```python
from build123d import *

# Parameters (mm, degrees)
BOSS_EXTRUDE1_START = -4
BOSS_EXTRUDE1_DEPTH = 8
CUT_EXTRUDE1_START  = -8
CUT_EXTRUDE1_DEPTH  = 6.4
CUT_EXTRUDE2_DEPTH  = 22.959710978
FILLET1_R           = 2.54
SKETCH6_R           = 3.25
CUT_EXTRUDE5_DEPTH  = 6.80625
LPATTERN1_COUNT     = 4
LPATTERN1_PITCH     = 8
SKETCH4_R           = 1.651
CUT_EXTRUDE3_DEPTH  = 36.358576134
SKETCH5_R           = 3.175
CUT_EXTRUDE4_DEPTH  = 2.54


# Read off the part's stored shape, not the designer's step: Boss-Extrude1
with BuildPart() as part:
    # Boss-Extrude1 outline → Boss-Extrude1 (new body)
    with BuildSketch(Plane(origin=(0, 0, 0), x_dir=(1, 0, 0), z_dir=(0, 1, 0)).offset(BOSS_EXTRUDE1_START)):
        Polygon((0, -4.7625), (0, 0), (-7.9375, 0), (-7.9375, 12.7), (-17.4625, 12.7), (-17.4625, -4.7625), align=None)
    extrude(amount=BOSS_EXTRUDE1_DEPTH)

    # Sketch2 → Cut-Extrude1 (cut)
    with BuildSketch(Plane(origin=(0, 0, -12.7), x_dir=(-1, 0, 0), z_dir=(0, 0, -1)).offset(CUT_EXTRUDE1_START)):
        with BuildLine():
            Line((17.4625, -3.1), (12.625, -3.1))
            ThreePointArc((12.625, -3.1), (9.525, 0), (12.625, 3.1))
            Line((12.625, 3.1), (17.4625, 3.1))
            ThreePointArc((17.4625, 3.1), (20.5625, 0), (17.4625, -3.1))
        make_face()
    extrude(amount=-CUT_EXTRUDE1_DEPTH, mode=Mode.SUBTRACT)

    # Sketch3 → Cut-Extrude2 (cut, through all)
    with BuildSketch(Plane.ZY.offset(17.4625)):
        with BuildLine():
            Line((-12.7, 0.79375), (-5.89375, 0.79375))
            ThreePointArc((-5.89375, 0.79375), (-5.1, 0), (-5.89375, -0.79375))
            Line((-5.89375, -0.79375), (-12.7, -0.79375))
            ThreePointArc((-12.7, -0.79375), (-13.49375, 0), (-12.7, 0.79375))
        make_face()
    extrude(amount=-CUT_EXTRUDE2_DEPTH, mode=Mode.SUBTRACT)

    # Fillet1
    fillet1_edges = [part.edges().sort_by_distance(p)[0] for p in [
        (-7.9375, 0, 0),
    ]]
    fillet(fillet1_edges, radius=FILLET1_R)

    # Sketch6 → Cut-Extrude5 (cut)
    with BuildSketch(Plane(origin=(0, 0, -12.7), x_dir=(-1, 0, 0), z_dir=(0, 0, -1))):
        with Locations((12.7, 0)):
            Circle(SKETCH6_R)
    extrude(amount=-CUT_EXTRUDE5_DEPTH, mode=Mode.SUBTRACT)

    # Mirror1: part across plane


with BuildPart() as part_1:
    add(part.part)
    add(part.part.mirror(Plane(origin=(0, 4, 0), x_dir=(0, 0, 1), z_dir=(-1, 0, 0))))


with BuildPart() as lpattern1_1:
    # LPattern1: pattern copy
    add(part_1.part.moved(Location(Vector(0, -1, 0) * (1 * LPATTERN1_PITCH))))


with BuildPart() as lpattern1_2:
    # LPattern1: pattern copy
    add(part_1.part.moved(Location(Vector(0, -1, 0) * (2 * LPATTERN1_PITCH))))


with BuildPart() as lpattern1_3:
    # LPattern1: pattern copy
    add(part_1.part.moved(Location(Vector(0, -1, 0) * (3 * LPATTERN1_PITCH))))


with BuildPart() as part_2:
    add(part_1.part)

    # Combine1: union LPattern1_1, LPattern1_2, LPattern1_3
    add(lpattern1_1.part)
    add(lpattern1_2.part)
    add(lpattern1_3.part)

    # Sketch4 → Cut-Extrude3 (cut, through all)
    with BuildSketch(Plane(origin=(0, 0, 0), x_dir=(-1, 0, 0), z_dir=(0, 0, -1))):
        Circle(SKETCH4_R)
        with Locations((0, -24)):
            Circle(SKETCH4_R)
    extrude(amount=-CUT_EXTRUDE3_DEPTH, mode=Mode.SUBTRACT)

    # Sketch5 → Cut-Extrude4 (cut)
    with BuildSketch(Plane(origin=(0, 0, 0), x_dir=(-1, 0, 0), z_dir=(0, 0, -1))):
        Circle(SKETCH5_R)
        with Locations((0, -24)):
            Circle(SKETCH5_R)
    extrude(amount=-CUT_EXTRUDE4_DEPTH, mode=Mode.SUBTRACT)


solid = part_2.part
```
CAD build for the part. Positions are in the model's coordinates, mm. A direction names the side the tool comes from. Round coordinates to 2 decimals unless told otherwise and drop trailing zeros. Loops run counter-clockwise (first coordinate to the right, second up) from the corner with the lowest first, then second, coordinate; pieces in that order, holes last. Notation, with made-up numbers: M 25,-9.75 L 38,-9.75 A21 cw 38,-4.75 Z; hole C -7.5,8 d3. An arc over 180 degrees is marked long. Return JSON: item names as keys, results as strings. Group by question number.
(1) Tool access for faces 4 (the cylindrical face through (-12.76, -4.75, -9.34)), 5 (the flat face through (-15, -12.9, -2)), 6 (the flat face through (-9, -15.206, -9)): list every direction of +Z, -Z, +X, -X, +Y, -Y with a clear straight run to the whole face (end or side of a thin tool).
(2) Mould opens along Z. For faces 1 (the flat face through (12.6, 3.4, -12.7)), 2 (the flat face through (17, -0.794, -9)), 3 (the flat face through (-15, -27.1, -2)) say: +Z half, -Z half, draft (parallel to the pull), parting line (faces both ways), or undercut.
(3) Wall check: probe 1 along Y at (x, z) = (0, 3.5); probe 2 along Y at (x, z) = (0, 0.65) (3 decimals); probe 3 along Y at (x, z) = (15, -4.5). Give the ranges that are in metal, low to high. Write a range as [from, to].
(4) Drop flat-ended pins along their axis: P1, Ø1.9, axis at x = 12, y = 0, coming from the -Z side; P2, Ø1.5, axis at y = -8, z = -3, coming from the -X side; P3, Ø3, axis at x = -3, y = -23.5, coming from the -Z side. Give the stop position or say it passes through.
(5) Saw through at C-C, the plane z = -7.5. Give the number of separate pieces and of enclosed holes in the cut face, and give its area (3 significant figures).
(6) Saw through at B-B, the plane y = -24. List the corners of the cut face in (x, z) (1 decimal).
(7) Saw through at A-A, the plane x = 0. List the corners of the cut face in (y, z) (1 decimal), and give its area (3 significant figures).
(8) Saw through at D-D, the plane y = -16. List the corners of the cut face in (x, z) (1 decimal), and give its area (3 significant figures).
Answer list:
{
 "1": {"face 4": "-Z", "face 5": "-X", "face 6": "-Z, +X, -X"},
 "2": {"face 1": "-Z half", "face 2": "draft", "face 3": "undercut"},
 "3": {"probe 1": "[-28, -25.65], [-22.35, -1.65], [1.65, 4]", "probe 2": "[-28, -27.175], [-20.825, -3.175], [3.175, 4]", "probe 3": "[-28, -27.1], [-20.9, -19.1], [-12.9, -11.1], [-4.9, -3.1], [3.1, 4]"},
 "4": {"P1": "z = -5.89", "P2": "x = -9.62", "P3": "z = 0"},
 "5": {"separate pieces": "10", "enclosed holes": "0", "area": "305 mm2"},
 "6": {"outline": "M -17.5,-5.1 L -7.9,-5.1 L -7.9,-2.5 A2.5 cw -5.4,0 L -3.2,0 L -3.2,2.5 L -1.7,2.5 L -1.7,4.8 L -17.5,4.8 L -17.5,1.7 L -9.5,1.7 L -9.5,-4.7 L -17.5,-4.7 Z; M 1.7,2.5 L 3.2,2.5 L 3.2,0 L 5.4,0 A2.5 cw 7.9,-2.5 L 7.9,-5.1 L 17.5,-5.1 L 17.5,-4.7 L 9.5,-4.7 L 9.5,1.7 L 17.5,1.7 L 17.5,4.8 L 1.7,4.8 Z"},
 "7": {"outline": "M -28,0 L -27.2,0 L -27.2,2.5 L -25.7,2.5 L -25.7,4.8 L -28,4.8 Z; M -22.3,2.5 L -20.8,2.5 L -20.8,0 L -3.2,0 L -3.2,2.5 L -1.7,2.5 L -1.7,4.8 L -22.3,4.8 Z; M 1.7,2.5 L 3.2,2.5 L 3.2,0 L 4,0 L 4,4.8 L 1.7,4.8 Z", "area": "105 mm2"},
 "8": {"outline": "M -17.5,-5.1 L -7.9,-5.1 L -7.9,-2.5 A2.5 cw -5.4,0 L 5.4,0 A2.5 cw 7.9,-2.5 L 7.9,-5.1 L 17.5,-5.1 L 17.5,-4.7 L 9.5,-4.7 L 9.5,1.7 L 17.5,1.7 L 17.5,4.8 L -17.5,4.8 L -17.5,1.7 L -9.5,1.7 L -9.5,-4.7 L -17.5,-4.7 Z", "area": "165 mm2"}
}
